from build123d import *

# Parameters (mm, degrees)
BOSS_EXTRU_1_DEPTH           = 40
ENL_V_MAT_EXTRU_1_DEPTH      = 76.498344353
ENL_V_MAT_EXTRU_1_DEPTH_BACK = 76.498344353
ESQUISSE2_R                  = 2.25
ENL_V_MAT_EXTRU_2_DEPTH      = 76.498344353
ENL_V_MAT_EXTRU_2_DEPTH_BACK = 76.498344353
ESQUISSE3_R                  = 2.25
ENL_V_MAT_EXTRU_3_DEPTH      = 96.640449297
ENL_V_MAT_EXTRU_3_DEPTH_BACK = 20
ESQUISSE4_R                  = 2.1
BOSS_EXTRU_2_DEPTH           = 4
BOSS_EXTRU_3_START           = -40
BOSS_EXTRU_3_DEPTH           = 4
BOSS_EXTRU_4_DEPTH           = 3
BOSS_EXTRU_4_DEPTH_BACK      = 3
BOSS_EXTRU_4_START           = -20


with BuildPart() as part:
    # Esquisse1 → Boss.-Extru.1 (new body)
    with BuildSketch(Plane(origin=(0, 0, 0), x_dir=(0, 0, -1), z_dir=(1, 0, 0))):
        Polygon((0, 0), (40, 0), (40, 10), (0, 10), (0, 36), (-15, 36), (-35, 1.358983849), (-20, -7.301270189), (-10, -7.301270189), (-10, -40), (0, -40), align=None)
    extrude(amount=BOSS_EXTRU_1_DEPTH)

    # Esquisse2 → Enlèv. mat.-Extru.1 (cut, two sides: drawn at the far end of the back side and taken through both)
    with BuildSketch(Plane(origin=(0, 10, 0), x_dir=(1, 0, 0), z_dir=(0, 1, 0)).offset(-ENL_V_MAT_EXTRU_1_DEPTH_BACK)):
        with Locations(Location((10, 30, 0), (0, 0, 270))):
            Circle(ESQUISSE2_R)
        with Locations(Location((30, 30, 0), (0, 0, 270))):
            Circle(ESQUISSE2_R)
        with Locations(Location((30, 10, 0), (0, 0, 270))):
            Circle(ESQUISSE2_R)
        with Locations(Location((10, 10, 0), (0, 0, 270))):
            Circle(ESQUISSE2_R)
    extrude(amount=ENL_V_MAT_EXTRU_1_DEPTH + ENL_V_MAT_EXTRU_1_DEPTH_BACK, mode=Mode.SUBTRACT)

    # Esquisse3 → Enlèv. mat.-Extru.2 (cut, two sides: drawn at the far end of the back side and taken through both)
    with BuildSketch(Plane.XY.offset(10).offset(-ENL_V_MAT_EXTRU_2_DEPTH_BACK)):
        with Locations((10, -33.650635095)):
            Circle(ESQUISSE3_R)
        with Locations((30, -33.650635095)):
            Circle(ESQUISSE3_R)
        with Locations((30, -13.650635095)):
            Circle(ESQUISSE3_R)
        with Locations((10, -13.650635095)):
            Circle(ESQUISSE3_R)
    extrude(amount=ENL_V_MAT_EXTRU_2_DEPTH + ENL_V_MAT_EXTRU_2_DEPTH_BACK, mode=Mode.SUBTRACT)

    # Esquisse4 → Enlèv. mat.-Extru.3 (cut, two sides: drawn at the far end of the back side and taken through both)
    with BuildSketch(Plane(origin=(0, 15.495190528, 26.838457268), x_dir=(1, 0, 0), z_dir=(0, 0.4999999999999946, 0.8660254037844419)).offset(-ENL_V_MAT_EXTRU_3_DEPTH_BACK)):
        with Locations(Location((20, 13.676914536, 0), (0, 0, 90))):
            Circle(ESQUISSE4_R)
        with Locations(Location((20, -6.323085464, 0), (0, 0, 90))):
            Circle(ESQUISSE4_R)
    extrude(amount=ENL_V_MAT_EXTRU_3_DEPTH + ENL_V_MAT_EXTRU_3_DEPTH_BACK, mode=Mode.SUBTRACT)

    # Esquisse5 → Boss.-Extru.2 (add)
    with BuildSketch(Plane(origin=(40, 0, 0), x_dir=(0, 0, -1), z_dir=(1, 0, 0))):
        Polygon((40, 10), (0, 36), (0, 10), align=None)
    extrude(amount=-BOSS_EXTRU_2_DEPTH)

    # Esquisse5<2> → Boss.-Extru.3 (add)
    with BuildSketch(Plane(origin=(40, 0, 0), x_dir=(0, 0, -1), z_dir=(1, 0, 0)).offset(BOSS_EXTRU_3_START)):
        Polygon((40, 10), (0, 36), (0, 10), align=None)
    extrude(amount=BOSS_EXTRU_3_DEPTH)

    # Esquisse5<3> → Boss.-Extru.4 (add, two sides: drawn at the far end of the back side and taken through both)
    with BuildSketch(Plane(origin=(40, 0, 0), x_dir=(0, 0, -1), z_dir=(1, 0, 0)).offset(BOSS_EXTRU_4_START - BOSS_EXTRU_4_DEPTH_BACK)):
        Polygon((40, 10), (0, 36), (0, 10), align=None)
    extrude(amount=BOSS_EXTRU_4_DEPTH + BOSS_EXTRU_4_DEPTH_BACK)


solid = part.part
Verification items for the finished model (mm, model axes). A direction names the side the tool comes from. Give positions to 0.01 mm unless a question says otherwise; leave off trailing zeros. Order: outer loops, then holes, each group sorted by start corner. A loop starts at its lowest first (then second) coordinate and runs counter-clockwise, first axis right, second up. Notation, with made-up numbers: (-22.5, 19.5) -> (-11.5, 19.5) arc R18 cw to (-11.5, 35.5) -> close; hole circle Ø5 at (4, 3). An arc over 180 degrees is marked (long way). Answer as CSV lines item,"result".
Q1. Access from +Z, -Z, +X, -X, +Y, -Y to the whole of each face (thin tool, end or side, straight path). Record for faces 5 (the cylindrical face through (7.752, -13.552, 4.93)), 6 (the flat face through (10, 23, 0)), 7 (the flat face through (19.971, -0.006, 12.694)), 8 (the flat face through (20, 36, 7)), 9 (the flat face through (20, -23, 10)).
Solutions:
face 5,"+Z, -Z"
face 6,"-Z, +Y"
face 7,"none"
face 8,"+Z, -Z, +X, -X, +Y"
face 9,"+Z, +X, -X, -Y"
Q2. Scan lines: probe 1 along X at (y, z) = (2, -10); probe 2 along Y at (x, z) = (30, 8); probe 3 along Z at (x, y) = (10, 6). Record each from-to range of solid material in increasing order.
Solutions:
probe 1,"x = 0 to 7.75, 12.25 to 27.75, 32.25 to 40"
probe 2,"y = -40 to -35.9, -31.4 to -15.9, -11.4 to 36"
probe 3,"z = -40 to -32.25, -27.75 to -12.25, -7.75 to 32.32"
Q3. Sectioned sample at D-D on y = -24. Record the cut outline in (x, z).
Solutions:
outline,"(0, 0) -> (40, 0) -> (40, 10) -> (0, 10) -> close"
Q4. Sectioned sample at A-A on z = -30. Record the cut outline in (x, y), plus the area to 3 significant figures.
Solutions:
outline,"(0, 0) -> (7.75, 0) -> (7.75, 10) -> (4, 10) -> (4, 16.5) -> (0, 16.5) -> close; (12.25, 0) -> (27.75, 0) -> (27.75, 10) -> (23, 10) -> (23, 16.5) -> (17, 16.5) -> (17, 10) -> (12.25, 10) -> close; (32.25, 0) -> (40, 0) -> (40, 16.5) -> (36, 16.5) -> (36, 10) -> (32.25, 10) -> close"
area,"401 mm²"
Q5. Sectioned sample at B-B on x = 30. Record the cut outline in (y, z), plus the area to 3 significant figures.
Solutions:
outline,"(-40, 0) -> (-35.9, 0) -> (-35.9, 10) -> (-40, 10) -> close; (-31.4, 0) -> (-15.9, 0) -> (-15.9, 10) -> (-31.4, 10) -> close; (-11.4, 0) -> (0, 0) -> (0, -7.75) -> (10, -7.75) -> (10, 0) -> (36, 0) -> (36, 15) -> (1.36, 35) -> (-7.3, 20) -> (-7.3, 10) -> (-11.4, 10) -> close; (0, -40) -> (10, -40) -> (10, -32.25) -> (0, -32.25) -> close; (0, -27.75) -> (10, -27.75) -> (10, -12.25) -> (0, -12.25) -> close"
area,"1,650 mm²"
Q6. Sectioned sample at C-C on z = -6. Record the cut outline in (x, y).
Solutions:
outline,"(0, 0) -> (40, 0) -> (40, 32.1) -> (36, 32.1) -> (36, 10) -> (23, 10) -> (23, 32.1) -> (17, 32.1) -> (17, 10) -> (4, 10) -> (4, 32.1) -> (0, 32.1) -> close"
Q7. Depth check by flat-ended pin: pin 1 (3 mm diameter, centred on x = 13, y = -17, fed in from -Z); pin 2 (3 mm diameter, centred on x = 26.5, z = 18.5, fed in from +Y); pin 3 (6 mm diameter, centred on x = 10, y = -13.65, fed in from +Z); pin 4 (3.5 mm diameter, centred on x = 30, z = -10, fed in from +Y). Enter the tip coordinate at first touch or a pass-through.
Solutions:
pin 1,"stops at z = 0"
pin 2,"stops at y = 32.54"
pin 3,"stops at z = 10"
pin 4,"passes through"
Q8. Release check for a two-part mould opening along Y. For faces 1 (the cylindrical face through (32.08, -14.51, 4.93)), 2 (the cylindrical face through (31.038, -35.647, 4.93)), 3 (the flat face through (20, -7.301, 15)), 4 (the flat face through (40, 7, -2)) record: +Y half, -Y half, draft (parallel to the pull), parting line (faces both ways), or undercut.
Solutions:
face 1,"undercut"
face 2,"undercut"
face 3,"-Y half"
face 4,"draft"
